CAD build for the part. Positions are in the model's coordinates, mm. A direction names the side the tool comes from. Round coordinates to 2 decimals unless told otherwise and drop trailing zeros. Write each loop counter-clockwise with the first axis right and the second up, starting at its lowest first coordinate (ties: lowest second). Pieces come first, ordered by that corner, then holes. Notation, with made-up numbers: (0, 71.25) - (30, 71.25) arc R23 ccw to (30, 89.25) - close; hole circle Ø2 at (83.25, 26). An arc over 180 degrees is marked (long way). Answer in a Markdown table with one row per item.
```python
from build123d import *

# Parameters (mm, degrees)
F0_W     = 18.5
F0_H     = 9
F1_DEPTH = 1
F2_W     = 15.5
F2_H     = 6
F3_DEPTH = 1
F4_R     = 1.975
F4_W     = 3
F4_H     = 2
F5_DEPTH = 2


with BuildPart() as f1:
    # F0 (on Top) → F1 (new body)
    with BuildSketch(Plane.XY):
        Rectangle(F0_W, F0_H)
    extrude(amount=F1_DEPTH)

    # F2 (on face) → F3 (join)
    with BuildSketch(Plane.XY.offset(1)):
        Rectangle(F2_W, F2_H)
    extrude(amount=F3_DEPTH)

    # F4 (on face) → F5 (cut)
    with BuildSketch(Plane.XY.offset(2)):
        Circle(F4_R)
        with Locations((-6.25, -2)):
            Rectangle(F4_W, F4_H)
    extrude(amount=-F5_DEPTH, mode=Mode.SUBTRACT)


solid = f1.part
```
Q1. 3-axis set-ups, long thin cutter, end or side, ignore diameter. For faces 5 (the flat face through (-7.75, 1, 1.5)), 6 (the flat face through (7.75, 0, 1.5)), 7 (the flat face through (1.4, -3, 1.5)), 8 (the flat face through (-7.75, -2, 0.5)): which of +Z, -Z, +X, -X, +Y, -Y reach the whole face in a straight line?
Computed:
| item | result |
|---|---|
| face 5 | +Z, -X, +Y, -Y |
| face 6 | +Z, +X, +Y, -Y |
| face 7 | +Z, +X, -X, -Y |
| face 8 | +Z, -Z |
Q2. Saw through at D-D on x = -2.75. List the corners of the cut face in (y, z).
Computed:
| item | result |
|---|---|
| outline | (-4.5, 0) - (4.5, 0) - (4.5, 1) - (3, 1) - (3, 2) - (-3, 2) - (-3, 1) - (-4.5, 1) - close |
Q3. Pull direction X, two halves, no side cores. Call faces 1 (the flat face through (-0.1, 4.5, 0.5)), 2 (the flat face through (-4.75, -2, 1)), 3 (the flat face through (-6, -1, 1)), 4 (the flat face through (-9.25, -0.1, 0.5)): released by +X, released by -X, zero draft, split by the parting line, or undercut.
Computed:
| item | result |
|---|---|
| face 1 | zero draft |
| face 2 | undercut |
| face 3 | undercut |
| face 4 | released by -X |
Q4. Drill centre lines: line 1 (Y direction, x = 0, z = 1.55) (3 decimals); line 2 (Y direction, x = -5, z = 1.4); line 3 (Y direction, x = -3, z = 1.2). Where is each one in solid material? Low to high.
Computed:
| item | result |
|---|---|
| line 1 | y = -3 to -1.975, 1.975 to 3 |
| line 2 | y = -1 to 3 |
| line 3 | y = -3 to 3 |
Q5. Saw through at C-C on z = 1.3. List the corners of the cut face in (x, y) (3 decimals), then the cut area to 3 significant figures.
Computed:
| item | result |
|---|---|
| outline | (-7.75, -1) - (-4.75, -1) - (-4.75, -3) - (7.75, -3) - (7.75, 3) - (-7.75, 3) - close; hole circle Ø3.95 at (0, 0) |
| area | 74.7 mm2 |
Q6. Saw through at B-B on y = 0. List the corners of the cut face in (x, z) (3 decimals).
Computed:
| item | result |
|---|---|
| outline | (-9.25, 0) - (-1.975, 0) - (-1.975, 2) - (-7.75, 2) - (-7.75, 1) - (-9.25, 1) - close; (1.975, 0) - (9.25, 0) - (9.25, 1) - (7.75, 1) - (7.75, 2) - (1.975, 2) - close |
Q7. Flat gauge pins, fed straight in: pin 1 (0.8 mm diameter, centred on y = -1, z = 1.5, fed in from +X); pin 2 (3 mm diameter, centred on x = 1.5, y = 2.5, fed in from -Z). Where does each tip first touch, or does it go through?
Computed:
| item | result |
|---|---|
| pin 1 | stops at x = 7.75 |
| pin 2 | stops at z = 0 |
Q8. Saw through at A-A on x = 0. List the corners of the cut face in (y, z) (3 decimals).
Computed:
| item | result |
|---|---|
| outline | (-4.5, 0) - (-1.975, 0) - (-1.975, 2) - (-3, 2) - (-3, 1) - (-4.5, 1) - close; (1.975, 0) - (4.5, 0) - (4.5, 1) - (3, 1) - (3, 2) - (1.975, 2) - close |
